The model under review builds one solid part; all positions refer to its coordinate system, in mm. A direction names the side the tool comes from. Give positions to 0.01 mm unless a question says otherwise; leave off trailing zeros. Loops run counter-clockwise (first coordinate to the right, second up) from the corner with the lowest first, then second, coordinate; pieces in that order, holes last. Notation, with made-up numbers: M 15,53 L 46,53 A14 ccw 46,73 Z; hole C 33.25,18.5 d4. An arc over 180 degrees is marked long. Put each result on its own line as item: value. Start each with the question number.
```python
from build123d import *

# Parameters (mm, degrees)
SKETCH_1_R      = 11
SKETCH_1_W      = 13
SKETCH_1_H      = 3
EXTRUDE_1_DEPTH = 3
FILLET_1_R      = 7
CHAMFER_1_SIZE  = 1


with BuildPart() as part:
    # 草图1 → 凸台-拉伸1 (new body)
    with BuildSketch(Plane(origin=(0, 0, 0), x_dir=(0, 0, -1), z_dir=(1, 0, 0))):
        with BuildLine():
            Line((13, 6.1), (-13, 6.1))
            Line((-13, 6.1), (-13, 2.01))
            ThreePointArc((-13, 2.01), (-12.289357685, 1.715642315), (-11.995, 1.005))
            ThreePointArc((-11.995, 1.005), (-12.289357685, 0.294357685), (-13, 0))
            Line((-13, 0), (-16.5, 0))
            Line((-16.5, 0), (-16.5, -8))
            Line((-16.5, -8), (-13, -8))
            ThreePointArc((-13, -8), (-12.289357685, -8.294357685), (-11.995, -9.005))
            ThreePointArc((-11.995, -9.005), (-12.289357685, -9.715642315), (-13, -10.01))
            Line((-13, -10.01), (-13, -12.733500839))
            ThreePointArc((-13, -12.733500839), (-11.507561308, -39.952303338), (8.174286015, -21.091882644))
            Line((8.174286015, -21.091882644), (13, -12.733500839))
            Line((13, -12.733500839), (13, -10.01))
            ThreePointArc((13, -10.01), (11.995, -9.005), (13, -8))
            Line((13, -8), (16.5, -8))
            Line((16.5, -8), (16.5, 0))
            Line((16.5, 0), (13, 0))
            ThreePointArc((13, 0), (11.995, 1.005), (13, 2.01))
            Line((13, 2.01), (13, 6.1))
        make_face()
        with Locations((-6, -26)):
            Circle(SKETCH_1_R, mode=Mode.SUBTRACT)
        with Locations((0, -8.6)):
            Rectangle(SKETCH_1_W, SKETCH_1_H, mode=Mode.SUBTRACT)
        with BuildLine():
            Line((5.59, -3.1), (-5.59, -3.1))
            ThreePointArc((-5.59, -3.1), (-6.595, -4.105), (-7.6, -3.1))
            Line((-7.6, -3.1), (-7.6, 1.09))
            ThreePointArc((-7.6, 1.09), (-8.605, 2.095), (-7.6, 3.1))
            Line((-7.6, 3.1), (7.6, 3.1))
            ThreePointArc((7.6, 3.1), (8.310642315, 2.805642315), (8.605, 2.095))
            ThreePointArc((8.605, 2.095), (8.310642315, 1.384357685), (7.6, 1.09))
            Line((7.6, 1.09), (7.6, -3.1))
            ThreePointArc((7.6, -3.1), (6.595, -4.105), (5.59, -3.1))
        make_face(mode=Mode.SUBTRACT)
    extrude(amount=EXTRUDE_1_DEPTH)

    # 圆角1
    fillet_1_edges = [part.edges().sort_by_distance(p)[0] for p in [
        (1.5, -21.091882644, -8.174286015),
    ]]
    fillet(fillet_1_edges, radius=FILLET_1_R)

    # 倒角1
    chamfer_1_edges = [part.edges().sort_by_distance(p)[0] for p in [
        (1.5, 6.1, 13),
        (1.5, 6.1, -13),
    ]]
    chamfer(chamfer_1_edges, length=CHAMFER_1_SIZE)


solid = part.part
```
Item 1: Consider section A-A, the plane y = -26. Write out the cut boundary in (x, z), plus the area to 3 significant figures.
Item 2: Consider section C-C, the plane z = 16. Write out the cut boundary in (x, y).
Item 3: Consider section D-D, the plane x = 2.4. Give the number of separate pieces and of enclosed holes in the cut face, plus the area to 3 significant figures.
Item 4: To check wall thickness, follow L1, parallel to Y at x = 1.65, z = -5.5; L2, parallel to Y at x = 2.2, z = 6; L3, parallel to Z at x = 2.5, y = -3.5. State the ranges of each line that lie inside material, in increasing order. Write a range as [from, to].
Item 5: Consider section B-B, the plane z = 1. Write out the cut boundary in (x, y), plus the area to 3 significant figures.
Item 6: Clearance check with flat-ended pins moving along their axes: pin 1 Ø0.8 at (x, y) = (1.5, -11) entering from -Z; pin 2 Ø1.5 at (x, z) = (2.5, -12) entering from -Y; pin 3 Ø0.9 at (x, z) = (2, -15) entering from -Y. State where each tip first meets the part, or that it passes through.
Item 7: Draft analysis for pull direction Z (two halves, no side actions). For faces 6 (the flat face through (1, 3.1, 0)), 7 (the cylindrical face through (1.479, -4.105, 6.573)), 8 (the flat face through (3, -12, 3)), 9 (the flat face through (1.5, 5.6, 12.5)), state which applies: +Z half, -Z half, draft (parallel to the pull), parting line (faces both ways), or undercut.
Item 8: Tool access review of faces 1 (the flat face through (1, -8, 15)), 2 (the flat face through (1, 4, -13)), 3 (the flat face through (1, -9, -6.5)), 4 (the flat face through (1, -11, -13)), 5 (the flat face through (1, 4, 13)): name each direction out of +Z, -Z, +X, -X, +Y, -Y from which nothing blocks a thin tool from reaching the whole face with its end or side.
Report:
1. outline: M 0,-9 L 3,-9 L 3,-5 L 0,-5 Z; M 0,17 L 3,17 L 3,21 L 0,21 Z
1. area: 24.0 mm²
2. outline: M 0,-37.18 L 3,-37.18 L 3,-30.58 L 0,-30.58 Z; M 0,-21.42 L 3,-21.42 L 3,-14.82 L 0,-14.82 Z; M 0,-8 L 3,-8 L 3,0 L 0,0 Z
3. separate pieces: 1
3. enclosed holes: 3
3. area: 752 mm²
4. L1: [-35.63, -10.1], [-7.1, -3.1], [3.1, 6.1]
4. L2: [-41, -37], [-15, -10.1], [-7.1, -3.91], [3.1, 6.1]
4. L3: [-16.5, -7.52], [-5.67, 5.67], [7.52, 16.5]
5. outline: M 0,-40.14 L 3,-40.14 L 3,-35.8 L 0,-35.8 Z; M 0,-16.2 L 3,-16.2 L 3,-10.1 L 0,-10.1 Z; M 0,-7.1 L 3,-7.1 L 3,-3.1 L 0,-3.1 Z; M 0,3.1 L 3,3.1 L 3,6.1 L 0,6.1 Z
5. area: 52.3 mm²
6. pin 1: z = -13
6. pin 2: y = -15.76
6. pin 3: y = -8
7. face 6: undercut
7. face 7: undercut
7. face 8: draft
7. face 9: +Z half
8. face 1: +Z, +X, -X
8. face 2: -Z, +X, -X, +Y
8. face 3: +X, -X
8. face 4: -Z, +X, -X, -Y
8. face 5: +Z, +X, -X, +Y
